Autodesk Inventor part; units mm, degrees
ref_plane "YZ Plane" through (0, 0, 0) normal (1, 0, 0) x (0, 1, 0)
ref_plane "XZ Plane" through (0, 0, 0) normal (0, 1, 0) x (-1, 0, 0)
ref_plane "XY Plane" through (0, 0, 0) normal (0, 0, 1) x (1, 0, 0)
sketch "Skizze1" plane through (0, 0, 0) normal (0, 0, 1) x (1, 0, 0)
  line L0 (-0.7373, 6.915) -> (3, 6.915)
  line L1 (3, 6.915) -> (3, -6.915)
  line L2 (3, -6.915) -> (-3, -6.915)
  line L3 (-3, -6.915) -> (-3, 4.6523)
  line L4 (-3, 6.915) -> (3, -6.915) construction
  line L5 (3, 6.915) -> (-3, -6.915) construction
  line L6 (-3, 0) -> (3, 0)
  line L7 (1.925, 6) -> (1.925, 5.115)
  line L8 (0.625, 6) -> (0.625, 5.115)
  line L9 (-1.375, 5.115) -> (-1.375, 0)
  line L10 (0.625, 6) -> (1.925, 6)
  line L11 (-1.375, 5.115) -> (0.625, 5.115)
  line L12 (1.925, 5.115) -> (3, 5.115)
  line L13 (-3, 0) -> (3, 0)
  line L14 (0.625, -6) -> (0.625, -5.115)
  line L15 (-1.375, -5.115) -> (-1.375, 0)
  line L16 (0.625, -6) -> (1.925, -6)
  line L17 (-1.375, -5.115) -> (0.625, -5.115)
  line L18 (1.925, -5.115) -> (3, -5.115)
  line L19 (1.925, -5.115) -> (1.925, -6)
  line L20 (-3, 6.915) -> (2.008, 6.915) construction
  line L21 (-3, 6.915) -> (4, 6.915) construction
  line L22 (-3, 6.915) -> (-7.9497, 11.8647)
  line L23 (-3, 6.915) -> (4, 6.915) construction
  line L24 (-0.7373, 6.915) -> (-3.3906, 9.5683)
  line L25 (-4.5789, 6.2311) -> (-3, 4.6523)
  ellipse E0 centre (-8.3445, 11.8647) end of major axis (-7.059, 13.1503) minor radius 1.6987
  ellipse E1 centre (-8.3445, 11.8647) end of major axis (-6.4572, 13.7521) minor radius 2.3999
  arc A0 (-4.5682, 6.2204) -> (-8.6297, 9.3267) centre (-18.2185, -7.4192) ccw
  arc A1 (-5.8407, 12.5429) -> (-3.2355, 9.4133) centre (11.6468, 24.4506) ccw
  line L26 (-8.1548, 13.6227) -> (-10.1025, 11.6751)
  line L27 (-8.1548, 13.6227) -> (-8.3445, 14.3886)
  line L28 (-8.3445, 14.3886) -> (-10.8684, 11.8647)
  line L29 (-10.1025, 11.6751) -> (-10.8684, 11.8647)
  line L30 (-3, 4.6523) -> (-3, 6.915)
  line L31 (-3, 6.915) -> (-0.7373, 6.915)
  point P0 (0, 0)
  point P1 (1.925, 5.5575)
  point P2 (-8.5245, 12.4395)
  point P3 (3, -5.115)
  point P4 (1.275, -6)
  point P5 (1.275, 6)
  point P6 (2.4625, 5.115)
  point P7 (-5.4749, 9.3899)
  dimension "d34" = 1.6987
  dimension "d35" = 1.818
  dimension "d36" = 2.6691
  dimension "d37" = 2.4
  dimension "d0" = 6
  dimension "d19" = 1.3
  dimension "d20" = 2
  dimension "d26" = 1.8
  dimension "d27" = 1.8
  dimension "d30" = 135
  dimension "d40" = 12
  dimension "d41" = 0.885
  dimension "d44" = 7.2125
  dimension "d45" = 4.9497
  dimension "d46" = 4.7376
  dimension "d47" = 2.2627
extrude "Extrusion1" add sketch "Skizze1" along normal mid plane 15 contours L31 L22 E1 A1 L24 | L30 L25 A0 E1 L22 | E1 L29 E0 L22 | L22 E0 L27 E1
extrude "Extrusion2" add sketch "Skizze1" along normal mid plane 25 contours L0 L1 L12 L7 L10 L8 L11 L9 L6 L3 L30 L31 | L6 L15 L17 L14 L16 L19 L18 L1 L2 L3
sketch "Skizze2" plane through (-3, -6.915, -12.5) normal (-1, 0, 0) x (0, 0, 1)
  line L0 (2.5, 11.33) -> (22.5, 11.33)
  line L1 (22.5, 11.33) -> (22.5, 2.5)
  line L2 (22.5, 2.5) -> (2.5, 2.5)
  line L3 (2.5, 2.5) -> (2.5, 11.33)
  line L4 (2.5, 11.33) -> (22.5, 2.5) construction
  line L5 (22.5, 11.33) -> (2.5, 2.5) construction
  line L6 (0, 0) -> (0, 13.83)
  line L7 (0, 0) -> (25, 0)
  point P0 (12.5, 6.915)
  point P1 (12.5, 2.5)
  dimension "d50" = 2.5
  dimension "d51" = 2.5
extrude "Extrusion3" cut sketch "Skizze2" against normal up to surface (1.625 mm away)
properties part number "led-mount_3D-Druck"
Read the model definition and answer for the solid it produces. Units are mm, in the model's axes. A direction names the side the tool comes from. Coordinates: 2 decimals unless noted, no trailing zeros. Loops run counter-clockwise (first coordinate to the right, second up) from the corner with the lowest first, then second, coordinate; pieces in that order, holes last.
Q1. Which of the six approach directions +Z, -Z, +X, -X, +Y, -Y give full straight-line access (tool end or side, diameter ignored) to faces 4 (the face through (0.625, 5.6, -0.2)), 5 (the face through (-2, 0, 10)), 6 (the face through (0, 5.115, 0))?
Q2. Consider probe 1 along Y at (x, z) = (0.75, -8) (3 decimals); probe 2 along Z at (x, y) = (-1.5, -3.25); probe 3 along X at (y, z) = (-5.75, -1.75) (3 decimals). Determine where each line is inside the solid, lowest interval first.
Q3. The mould has two halves that part along Y. Classify faces 1 (the face through (3, 6, 0)), 2 (the face through (1, -6, 0)), 3 (the face through (0, -6.915, 0)): +Y half, -Y half, draft (parallel to the pull), parting line (faces both ways), or undercut.
Q4. The part is cut by section D-D on x = -2.25. Write down the section's boundary in (y, z) (3 decimals).
Q5. The part is cut by section A-A on z = -9.5. Write down the section's boundary in (x, y) (3 decimals), and give its area (3 significant figures).
Q6. Each of these flat-tipped pins is pushed along its axis until it touches: pin 1 Ø2 at (y, z) = (9, 3) entering from -X; pin 2 Ø1.7 at (x, y) = (-6.5, 8.5) entering from -Z; pin 3 Ø1.3 at (x, y) = (-9, 10.5) entering from +Z. Where does it stop, or does it pass through?
Q7. The part is cut by section B-B on y = -2.5. Write down the section's boundary in (x, z) (3 decimals).
Q8. The part is cut by section C-C on z = 10.5. Write down the section's boundary in (x, y) (3 decimals).
Results below:
1. face 4: +Z, -Z
1. face 5: +X, -X
1. face 6: +Z, -Z, +X
2. probe 1: y = -6.915 to -6, 6 to 6.915
2. probe 2: z = -12.5 to -10, 10 to 12.5
2. probe 3: x = -3 to 0.625, 1.925 to 3
3. face 1: draft
3. face 2: undercut
3. face 3: -Y half
4. outline: (-6.915, -12.5) - (6.915, -12.5) - (6.915, -7.5) - (8.428, -7.5) - (8.428, 7.5) - (6.915, 7.5) - (6.915, 12.5) - (-6.915, 12.5) - close; hole (-4.415, -10) - (4.415, -10) - (4.415, 10) - (-4.415, 10) - close
5. outline: (-3, -6.915) - (3, -6.915) - (3, -5.115) - (1.925, -5.115) - (1.925, -6) - (0.625, -6) - (0.625, -5.115) - (-1.375, -5.115) - (-1.375, -4.415) - (-3, -4.415) - close; (-3, 4.415) - (-1.375, 4.415) - (-1.375, 5.115) - (0.625, 5.115) - (0.625, 6) - (1.925, 6) - (1.925, 5.115) - (3, 5.115) - (3, 6.915) - (-3, 6.915) - close
5. area: 21.6 mm2
6. pin 1: stops at x = -10.25
6. pin 2: stops at z = -7.5
6. pin 3: stops at z = 7.5
7. outline: (-3, -12.5) - (-1.375, -12.5) - (-1.375, -10) - (-3, -10) - close; (-3, 10) - (-1.375, 10) - (-1.375, 12.5) - (-3, 12.5) - close
8. outline: (-3, -6.915) - (3, -6.915) - (3, -5.115) - (1.925, -5.115) - (1.925, -6) - (0.625, -6) - (0.625, -5.115) - (-1.375, -5.115) - (-1.375, 5.115) - (0.625, 5.115) - (0.625, 6) - (1.925, 6) - (1.925, 5.115) - (3, 5.115) - (3, 6.915) - (-3, 6.915) - close
